Input: part model. Units: mm. Frame: model coordinates. Coordinates: 2 decimals unless noted, no trailing zeros. Loops run counter-clockwise (first coordinate to the right, second up) from the corner with the lowest first, then second, coordinate; pieces in that order, holes last. Notation, with made-up numbers: (3, 66.25) -> (37, 66.25) arc R20 ccw to (37, 80.25) -> close; hole circle Ø1 at (38.25, -14). An arc over 180 degrees is marked (long way). Answer as a JSON object with one key per item and string values.
from build123d import *

# Parameters (mm, degrees)
F0_W     = 57.15
F0_H     = 31.75
F1_DEPTH = 25.4
F3_DEPTH = 25.4
F5_DEPTH = 25.4


with BuildPart() as f1:
    # F0 (on Front) → F1 (new body)
    with BuildSketch(Plane.XZ):
        with Locations((2.448356, 6.53348)):
            Rectangle(F0_W, F0_H)
    extrude(amount=F1_DEPTH)

    # F2 (on face) → F3 (cut)
    with BuildSketch(Plane.XZ.offset(25.4)):
        with BuildLine():
            Line((31.023356, 22.40848), (11.973356, 22.40848))
            ThreePointArc((11.973356, 22.40848), (17.552972, 8.938096), (31.023356, 3.35848))
            Line((31.023356, 3.35848), (31.023356, 22.40848))
        make_face()
    extrude(amount=-F3_DEPTH, mode=Mode.SUBTRACT)

    # F4 (on face) → F5 (cut)
    with BuildSketch(Plane.XZ.offset(25.4)):
        with BuildLine():
            ThreePointArc((-26.126644, 16.05848), (-24.244579, 20.526415), (-19.776644, 22.40848))
            Line((-19.776644, 22.40848), (-26.126644, 22.40848))
            Line((-26.126644, 22.40848), (-26.126644, 16.05848))
        make_face()
    extrude(amount=-F5_DEPTH, mode=Mode.SUBTRACT)


solid = f1.part
1. Line query: line 1 along Z through (x, y) = (-20, -2); line 2 along Z through (x, y) = (23, -9.25); line 3 along X through (y, z) = (-21.25, 13.5). Output: solid intervals per line, ascending.
Reply:
{"line 1": "z = -9.34 to 22.4", "line 2": "z = -9.34 to 5.13", "line 3": "x = -26.13 to 14.18"}
2. Pin query (flat end, axial travel): P1, Ø2, axis at y = -17, z = 11, coming from the +X side; P2, Ø1, axis at x = 14, y = -19, coming from the +Z side. Return the tip coordinate at first contact, or that it passes through.
Reply:
{"P1": "stops at x = 16.57", "P2": "stops at z = 14.94"}
3. Section query C-C (x = 13). Return loops of the section in (y, z), plus the area to 3 significant figures.
Reply:
{"outline": "(-25.4, -9.34) -> (0, -9.34) -> (0, 16.24) -> (-25.4, 16.24) -> close", "area": "650 mm2"}
4. Section query B-B (z = 7). Return loops of the section in (x, y).
Reply:
{"outline": "(-26.13, -25.4) -> (19.82, -25.4) -> (19.82, 0) -> (-26.13, 0) -> close"}
5. Section query A-A (y = -18.75). Return loops of the section in (x, z), plus the area to 3 significant figures.
Reply:
{"outline": "(-26.13, -9.34) -> (31.02, -9.34) -> (31.02, 3.36) arc R19.05 cw to (11.97, 22.41) -> (-19.78, 22.41) arc R6.43 ccw to (-26.13, 16.06) -> close", "area": "1,520 mm2"}
